Geometry check sheet. Reference: the model listing, model coordinates, mm. Face numbers are marked on the shaded views. A direction names the side the tool comes from. Coordinates: 2 decimals unless noted, no trailing zeros. Loops run counter-clockwise (first coordinate to the right, second up) from the corner with the lowest first, then second, coordinate; pieces in that order, holes last. Notation, with made-up numbers: (9.25, 29.25) - (63.25, 29.25) arc R32 cw to (63.25, 63.25) - close; hole circle Ø5 at (18.5, 85.5). An arc over 180 degrees is marked (long way). Write item = value, one per line. Start each with the question number.
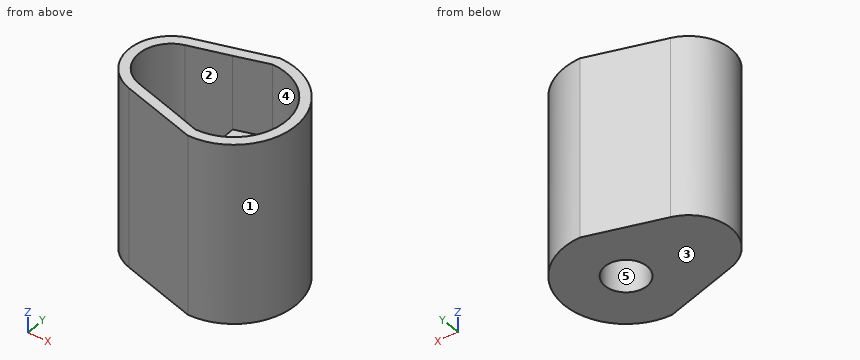
from build123d import *

# Parameters (mm, degrees)
F1_DEPTH  = 30
F3_DEPTH  = 27
F2_R      = 4
F5_DEPTH  = 6.5
F4_R      = 4.25
F4_R_2    = 4
F6_DEPTH  = 35.2
F7_DEPTH  = 10
F8_W      = 1
F8_H      = 16.5
F9_DEPTH  = 13.4
F11_DEPTH = 16
F12_DEPTH = 0.5
F13_R     = 1.25
F14_DEPTH = 25
F15_DEPTH = 2
F16_DEPTH = 18.5
F18_DEPTH = 15


with BuildPart() as f1:
    # F0 (on Top) → F1 (new body)
    with BuildSketch(Plane.XY):
        with BuildLine():
            ThreePointArc((-9.61, 7.9936162029), (-5.5424501439, 4.8828782496), (-4, 0))
            ThreePointArc((-4, 0), (-5.5424501439, -4.8828782496), (-9.61, -7.9936162029))
            ThreePointArc((-9.61, -7.9936162029), (-8.2636700449, -9.3787929602), (-6.72, -10.54))
            Line((-6.72, -10.54), (0, -12.5))
            ThreePointArc((0, -12.5), (8.8388347648, -8.8388347648), (12.5, 0))
            ThreePointArc((12.5, 0), (8.8388347648, 8.8388347648), (0, 12.5))
            Line((0, 12.5), (-6.72, 10.54))
            ThreePointArc((-6.72, 10.54), (-8.2636700449, 9.3787929602), (-9.61, 7.9936162029))
        make_face()
        with BuildLine():
            ThreePointArc((-4, 0), (0, 4), (4, 0))
            ThreePointArc((4, 0), (0, -4), (-4, 0))
        make_face(mode=Mode.SUBTRACT)
        with BuildLine():
            ThreePointArc((-9.61, -7.9936162029), (-5.5424501439, -4.8828782496), (-4, 0))
            ThreePointArc((-4, 0), (-5.5424501439, 4.8828782496), (-9.61, 7.9936162029))
            ThreePointArc((-9.61, 7.9936162029), (-12.5, 0), (-9.61, -7.9936162029))
        make_face()
        with BuildLine():
            ThreePointArc((-14.88, 8.16), (-12.231772686, 8.4957668346), (-9.61, 7.9936162029))
            ThreePointArc((-9.61, 7.9936162029), (-8.2636700449, 9.3787929602), (-6.72, 10.54))
            Line((-6.72, 10.54), (-14.88, 8.16))
        make_face()
        with BuildLine():
            ThreePointArc((-9.61, -7.9936162029), (-12.5, 0), (-9.61, 7.9936162029))
            ThreePointArc((-9.61, 7.9936162029), (-12.231772686, 8.4957668346), (-14.88, 8.16))
            ThreePointArc((-14.88, 8.16), (-21, 0), (-14.88, -8.16))
            ThreePointArc((-14.88, -8.16), (-12.231772686, -8.4957668346), (-9.61, -7.9936162029))
        make_face()
        with BuildLine():
            ThreePointArc((-6.72, -10.54), (-8.2636700449, -9.3787929602), (-9.61, -7.9936162029))
            ThreePointArc((-9.61, -7.9936162029), (-12.231772686, -8.4957668346), (-14.88, -8.16))
            Line((-14.88, -8.16), (-6.72, -10.54))
        make_face()
    extrude(amount=F1_DEPTH)

    # F2 (on face) → F3 (cut)
    with BuildSketch(Plane.XY.offset(30)):
        with BuildLine():
            Line((-14.32, -6.24), (-6.5, -8.5208333333))
            Line((-6.5, -8.5208333333), (-6.5, -6.5))
            Line((-6.5, -6.5), (-6.5, 6.5))
            Line((-6.5, 6.5), (-6.5, 8.5208333333))
            Line((-6.5, 8.5208333333), (-14.32, 6.24))
            ThreePointArc((-14.32, 6.24), (-19, 0), (-14.32, -6.24))
        make_face()
    extrude(amount=-F3_DEPTH, mode=Mode.SUBTRACT)

    # F2 (on face) → F5 (cut)
    with BuildSketch(Plane.XY.offset(30)):
        Polygon((-6.5, 6.5), (-6.5, -6.5), (6.5, -6.5), (10, 0), (6.5, 6.5), align=None)
        Circle(F2_R, mode=Mode.SUBTRACT)
    extrude(amount=-F5_DEPTH, mode=Mode.SUBTRACT)

    # F4 (on face) → F6 (cut)
    with BuildSketch(Plane.XY.offset(30)):
        Circle(F4_R)
        Circle(F4_R_2, mode=Mode.SUBTRACT)
    extrude(amount=-F6_DEPTH, mode=Mode.SUBTRACT)

    # F7 (add): a face of the model
    f7_faces = [f1.faces().sort_by_distance(p)[0] for p in [
        (-7.3229596651, 9.9287188517, 30),
    ]]
    extrude(f7_faces, amount=F7_DEPTH)

    # F8 (on face) → F9 (join)
    with BuildSketch(Plane.XZ.offset(-6.5)):
        with Locations((-6, 31.75)):
            Rectangle(F8_W, F8_H)
    extrude(amount=F9_DEPTH)

    # F10 (on face) → F11 (cut)
    with BuildSketch(Plane.XY.offset(40)):
        with BuildLine():
            Line((6.5, -6.5), (-5.5, -6.5))
            Line((-5.5, -6.5), (0, -12.5))
            ThreePointArc((0, -12.5), (12.5, 0), (0, 12.5))
            Line((0, 12.5), (-5.5, 6.5))
            Line((-5.5, 6.5), (6.5, 6.5))
            Line((6.5, 6.5), (10, 0))
            Line((10, 0), (6.5, -6.5))
        make_face()
    extrude(amount=-F11_DEPTH, mode=Mode.SUBTRACT)

    # F12 (cut): a face of the model
    f12_faces = [f1.faces().sort_by_distance(p)[0] for p in [
        (0.5, -6.808058436, 24),
    ]]
    extrude(f12_faces, amount=-F12_DEPTH, mode=Mode.SUBTRACT)

    # F13 (on face) → F14 (cut)
    with BuildSketch(Plane.YZ.offset(-5.5)):
        with Locations((0, 31.75)):
            Circle(F13_R)
    extrude(amount=-F14_DEPTH, mode=Mode.SUBTRACT)

    # F15 (cut): a face of the model
    f15_faces = [f1.faces().sort_by_distance(p)[0] for p in [
        (-2.5229134485, -9.2918373278, 23.5),
    ]]
    extrude(f15_faces, amount=-F15_DEPTH, mode=Mode.SUBTRACT)

    # F16 (cut): a face of the model
    f16_faces = [f1.faces().sort_by_distance(p)[0] for p in [
        (-2.9906782868, 9.7206217629, 40),
    ]]
    extrude(f16_faces, amount=-F16_DEPTH, mode=Mode.SUBTRACT)

    # F17 (on face) → F18 (join)
    with BuildSketch(Plane.XY.offset(21.5)):
        with BuildLine():
            ThreePointArc((-14.88, 8.16), (-21, 0), (-14.88, -8.16))
            Line((-14.88, -8.16), (0, -12.5))
            ThreePointArc((0, -12.5), (12.5, 0), (0, 12.5))
            Line((0, 12.5), (-14.88, 8.16))
        make_face()
        with BuildLine():
            ThreePointArc((0, 10.5), (10.5, 0), (0, -10.5))
            Line((0, -10.5), (-6.5, -8.5208333333))
            Line((-6.5, -8.5208333333), (-14.32, -6.24))
            ThreePointArc((-14.32, -6.24), (-19, 0), (-14.32, 6.24))
            Line((-14.32, 6.24), (-6.5, 8.5208333333))
            Line((-6.5, 8.5208333333), (0, 10.5))
        make_face(mode=Mode.SUBTRACT)
    extrude(amount=F18_DEPTH)


solid = f1.part
(1) Scan lines: line 1 (Y direction, x = 0, z = 8); line 2 (Z direction, x = -10, y = 4.25); line 3 (Z direction, x = -2, y = 7). Record each from-to range of solid material in increasing order.
(2) Sectioned sample at D-D on z = 15.5. Enter the section's corners in (x, y).
(3) Draft check along Y on the marked faces 1, 2 and 3. Enter one of: pulls with the +Y half, pulls with the -Y half, needs draft (parallel to the pull), parting line crosses it, or undercut.
(4) Sectioned sample at C-C on x = -0.5. Enter the section's corners in (y, z), plus the area to 3 significant figures.
(5) Sectioned sample at B-B on y = 0. Enter the section's corners in (x, z).
(6) Tool access check on the marked faces 4 and 5. Record the directions out of +Z, -Z, +X, -X, +Y, -Y that give a thin tool (end or side, any length) a straight path to the whole face; none if there is none.
(7) Depth check by flat-ended pin: pin 1 (1 mm diameter, centred on x = -16, y = -9.5, fed in from -Z); pin 2 (2 mm diameter, centred on x = 4, z = 32, fed in from -Y); pin 3 (8 mm diameter, centred on x = -8.5, z = 31.5, fed in from -Y); pin 4 (4 mm diameter, centred on y = 3, z = 31.5, fed in from +X). Enter the tip coordinate at first touch or a pass-through.
(8) Sectioned sample at A-A on z = 26.5. Enter the section's corners in (x, y), plus the area to 3 significant figures.
Working result:
q1.line_1 = -12.5 to -4.25, 4.25 to 12.5
q1.line_2 = 0 to 3
q1.line_3 = 0 to 21.5
q2.outline = (-14.88, -8.16) - (0, -12.5) arc R12.5 ccw to (0, 12.5) - (-14.88, 8.16) arc R8.5 ccw to start; hole (-14.32, -6.24) - (-6.5, -8.52) - (-6.5, 8.52) - (-14.32, 6.24) arc R6.5 ccw to start; hole circle Ø8.5 at (0, 0)
q3.face_1 = parting line crosses it
q3.face_2 = undercut
q3.face_3 = needs draft
q4.outline = (-12.35, 0) - (-4.22, 0) - (-4.22, 21.5) - (-10.35, 21.5) - (-10.35, 36.5) - (-12.35, 36.5) - close; (4.22, 0) - (12.35, 0) - (12.35, 36.5) - (10.35, 36.5) - (10.35, 21.5) - (4.22, 21.5) - close
q4.area = 410 mm2
q5.outline = (-21, 0) - (-4.25, 0) - (-4.25, 21.5) - (-6.5, 21.5) - (-6.5, 3) - (-19, 3) - (-19, 36.5) - (-21, 36.5) - close; (4.25, 0) - (12.5, 0) - (12.5, 36.5) - (10.5, 36.5) - (10.5, 21.5) - (4.25, 21.5) - close
q6.face_4 = +Z
q6.face_5 = +Z, -Z
q7.pin_1 = through
q7.pin_2 = -12.13
q7.pin_3 = -11.19
q7.pin_4 = 12.46
q8.outline = (-14.88, -8.16) - (0, -12.5) arc R12.5 ccw to (0, 12.5) - (-14.88, 8.16) arc R8.5 ccw to start; hole (-14.32, -6.24) - (-6.5, -8.52) - (0, -10.5) arc R10.5 ccw to (0, 10.5) - (-6.5, 8.52) - (-14.32, 6.24) arc R6.5 ccw to start
q8.area = 171 mm2
